Could you check a few things on this drawing? It's one solid part, dimensions in mm from its lowest x, y, z. Coordinates: 2 decimals unless noted, no trailing zeros. Write each loop counter-clockwise with the first axis right and the second up, starting at its lowest first coordinate (ties: lowest second). Pieces come first, ordered by that corner, then holes.
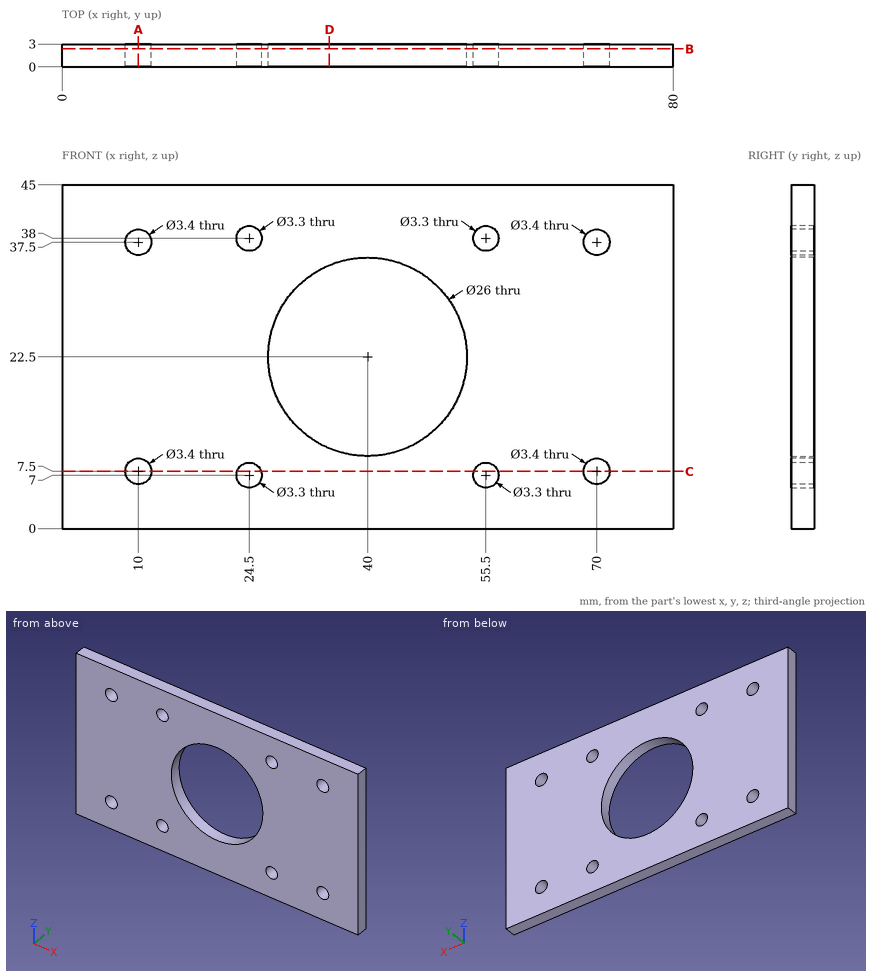
1) Imagine slicing it at D-D on x = 35. Please give me the cut outline in (y, z).
Values follow:
outline: (0, 0) - (3, 0) - (3, 10.5) - (0, 10.5) - close; (0, 34.5) - (3, 34.5) - (3, 45) - (0, 45) - close
2) Imagine slicing it at B-B on y = 2.35. Count the separate pieces of the cut face and the enclosed holes in it, then the cut area to 3 significant figures.
Values follow:
separate pieces: 1
enclosed holes: 9
area: 3,000 mm2
3) Will these pins go through, and if not, where does the flat tip stop? pin 1 (2 mm diameter, centred on x = 70, z = 7.5, fed in from -Y) (3 decimals); pin 2 (4 mm diameter, centred on x = 70, z = 37.5, fed in from -Y).
Values follow:
pin 1: passes through
pin 2: stops at y = 0
4) Imagine slicing it at C-C on z = 7.5. Please give me the cut outline in (x, y), then the cut area to 3 significant figures.
Values follow:
outline: (0, 0) - (8.3, 0) - (8.3, 3) - (0, 3) - close; (11.7, 0) - (22.93, 0) - (22.93, 3) - (11.7, 3) - close; (26.07, 0) - (53.93, 0) - (53.93, 3) - (26.07, 3) - close; (57.07, 0) - (68.3, 0) - (68.3, 3) - (57.07, 3) - close; (71.7, 0) - (80, 0) - (80, 3) - (71.7, 3) - close
area: 201 mm2
5) I need wall thicknesses on probe 1 along Z at (x, y) = (70, 1.9); probe 2 along Z at (x, y) = (10.5, 2.5); probe 3 along X at (y, z) = (2.1, 7.5). Which ranges of each line are inside material? Lowest first, please.
Values follow:
probe 1: z = 0 to 5.8, 9.2 to 35.8, 39.2 to 45
probe 2: z = 0 to 5.88, 9.12 to 35.88, 39.12 to 45
probe 3: x = 0 to 8.3, 11.7 to 22.93, 26.07 to 53.93, 57.07 to 68.3, 71.7 to 80
6) Imagine slicing it at A-A on x = 10. Please give me the cut outline in (y, z).
Values follow:
outline: (0, 0) - (3, 0) - (3, 5.8) - (0, 5.8) - close; (0, 9.2) - (3, 9.2) - (3, 35.8) - (0, 35.8) - close; (0, 39.2) - (3, 39.2) - (3, 45) - (0, 45) - close
